Check sheet for the modelled part. Datum: model origin and axes. Units: mm. A direction names the side the tool comes from. Round coordinates to 2 decimals unless told otherwise and drop trailing zeros. Order: outer loops, then holes, each group sorted by start corner. A loop starts at its lowest first (then second) coordinate and runs counter-clockwise, first axis right, second up.
Q1. Set-up check for faces 5 (the flat face through (-6.5, 0, 3)), 6 (the flat face through (-25.7, 7, 2)), 7 (the flat face through (28, -4, 2)), 8 (the flat face through (-28, -4, 2)): record each of +Z, -Z, +X, -X, +Y, -Y from which the full face is reachable in a straight line by a thin tool's end or side.
Q2. Depth check by flat-ended pin: P1, Ø2.5, axis at y = -6.5, z = 2, coming from the -X side; P2, Ø2.5, axis at x = -28, z = 2, coming from the -Y side; P3, Ø5, axis at x = 20, y = 4, coming from the -Z side; P4, Ø1.5, axis at y = -8, z = 3, coming from the +X side. Enter the tip coordinate at first touch or a pass-through.
Q3. Cross-section at B-B on z = 3.25. Record the cut outline in (x, y).
Q4. Mould release check, pull along X, two halves, no side actions. Record for faces 1 (the flat face through (-25.7, -7, 2)), 2 (the flat face through (0, -4, 3)), 3 (the flat face through (25.7, -7, 2)), 4 (the flat face through (28, 4, 2)): +X half, -X half, draft (parallel to the pull), parting line (faces both ways), or undercut.
Q5. Scan lines: probe 1 along Y at (x, z) = (-4, 0.9); probe 2 along X at (y, z) = (-3.25, 2.5); probe 3 along X at (y, z) = (6.5, 0.45). Record each from-to range of solid material in increasing order.
Q6. Cross-section at D-D on y = -5.75. Record the cut outline in (x, z).
Q7. Cross-section at C-C on x = 5.5. Record the cut outline in (y, z), then the cut area to 3 significant figures.
Q8. Cross-section at A-A on y = 1.5. Record the cut outline in (x, z), then the cut area to 3 significant figures.
from build123d import *

# Parameters (mm, degrees)
BOSS_EXTRUDE1_DEPTH = 5
SKETCH2_W           = 13
SKETCH2_H           = 8
CUT_EXTRUDE1_DEPTH  = 5


with BuildPart() as part:
    # Sketch1 → Boss-Extrude1 (new body)
    with BuildSketch(Plane.XY):
        Polygon((25.7, 10), (-25.7, 10), (-25.7, 4), (-31.2, 4), (-31.2, -4), (-25.7, -4), (-25.7, -10), (25.7, -10), (25.7, -4), (31.2, -4), (31.2, 4), (25.7, 4), align=None)
    extrude(amount=BOSS_EXTRUDE1_DEPTH)

    # Sketch2 → Cut-Extrude1 (cut)
    with BuildSketch(Plane.XY.offset(5)):
        Rectangle(SKETCH2_W, SKETCH2_H)
    extrude(amount=-CUT_EXTRUDE1_DEPTH, mode=Mode.SUBTRACT)


solid = part.part
Results found:
1. face 5: +Z, -Z
1. face 6: +Z, -Z, -X, +Y
1. face 7: +Z, -Z, +X, -Y
1. face 8: +Z, -Z, -X, -Y
2. P1: stops at x = -25.7
2. P2: stops at y = -4
2. P3: stops at z = 0
2. P4: stops at x = 25.7
3. outline: (-31.2, -4) - (-25.7, -4) - (-25.7, -10) - (25.7, -10) - (25.7, -4) - (31.2, -4) - (31.2, 4) - (25.7, 4) - (25.7, 10) - (-25.7, 10) - (-25.7, 4) - (-31.2, 4) - close; hole (-6.5, -4) - (6.5, -4) - (6.5, 4) - (-6.5, 4) - close
4. face 1: -X half
4. face 2: undercut
4. face 3: +X half
4. face 4: draft
5. probe 1: y = -10 to -4, 4 to 10
5. probe 2: x = -31.2 to -6.5, 6.5 to 31.2
5. probe 3: x = -25.7 to 25.7
6. outline: (-25.7, 0) - (25.7, 0) - (25.7, 5) - (-25.7, 5) - close
7. outline: (-10, 0) - (-4, 0) - (-4, 5) - (-10, 5) - close; (4, 0) - (10, 0) - (10, 5) - (4, 5) - close
7. area: 60.0 mm2
8. outline: (-31.2, 0) - (-6.5, 0) - (-6.5, 5) - (-31.2, 5) - close; (6.5, 0) - (31.2, 0) - (31.2, 5) - (6.5, 5) - close
8. area: 247 mm2
